```python
from build123d import *

# Parameters (mm, degrees)
SKETCH1_W                       = 25.2476
SKETCH1_H                       = 29.5402
BOSS_EXTRUDE1_DEPTH             = 7.9502
CHAMFER1_SIZE                   = 0.762
CUT_EXTRUDE1_DEPTH              = 30.5402
F_4_40_TAPPED_HOLE1_D           = 2.2606
F_4_40_TAPPED_HOLE1_DEPTH       = 9.5504
F_4_40_TAPPED_HOLE1_CSINK_D     = 4.1148
F_4_40_TAPPED_HOLE1_CSINK_ANGLE = 90
F_4_40_TAPPED_HOLE1_TIP         = 0.679152758
SKETCH6_R                       = 1.6256
SKETCH6_W                       = 3.2512
SKETCH6_H                       = 12.7
CUT_EXTRUDE3_DEPTH              = 8.9502
CUT_EXTRUDE4_DEPTH              = 3.6322
SKETCH11_R                      = 0.635
CUT_EXTRUDE5_DEPTH              = 8.9502
CUT_EXTRUDE7_DEPTH              = 13.6238
CUT_EXTRUDE7_DEPTH_BACK         = 13.6238


with BuildPart() as part:
    # Sketch1 → Boss-Extrude1 (new body)
    with BuildSketch(Plane.XY):
        Rectangle(SKETCH1_W, SKETCH1_H)
    extrude(amount=BOSS_EXTRUDE1_DEPTH)

    # Chamfer1
    chamfer1_edges = [part.edges().sort_by_distance(p)[0] for p in [
        (12.6238, -14.7701, 3.9751),
        (-12.6238, -14.7701, 3.9751),
        (-12.6238, 14.7701, 3.9751),
        (12.6238, 14.7701, 3.9751),
    ]]
    chamfer(chamfer1_edges, length=CHAMFER1_SIZE)

    # Sketch2 → Cut-Extrude1 (cut, through all)
    with BuildSketch(Plane(origin=(0, 14.7701, 0), x_dir=(1, 0, 0), z_dir=(0, 1, 0))):
        Polygon((-6.35, 0.508), (-6.858, 0), (-6.35, -0.508), (-5.842, 0), align=None)
        Polygon((5.842, 0), (6.35, -0.508), (6.858, 0), (6.35, 0.508), align=None)
    extrude(amount=-CUT_EXTRUDE1_DEPTH, mode=Mode.SUBTRACT)

    # #4-40 Tapped Hole1
    with Locations(Plane(origin=(0, 14.7701, 0), x_dir=(1, 0, 0), z_dir=(0, 1, 0))):
        with Locations((-8.89, -3.81), (8.89, -3.81)):
            CounterSinkHole(F_4_40_TAPPED_HOLE1_D / 2, F_4_40_TAPPED_HOLE1_CSINK_D / 2, depth=F_4_40_TAPPED_HOLE1_DEPTH, counter_sink_angle=F_4_40_TAPPED_HOLE1_CSINK_ANGLE)
            with Locations((0, 0, -(F_4_40_TAPPED_HOLE1_DEPTH + F_4_40_TAPPED_HOLE1_TIP / 2))):  # 118° drill point
                Cone(0, F_4_40_TAPPED_HOLE1_D / 2, F_4_40_TAPPED_HOLE1_TIP, mode=Mode.SUBTRACT)

    # Sketch6 → Cut-Extrude3 (cut, through all)
    with BuildSketch(Plane.XY.offset(7.9502)):
        with Locations((-6.35, 0.6985)):
            Circle(SKETCH6_R)
        with Locations((-6.35, -12.0015)):
            Circle(SKETCH6_R)
        with Locations((6.35, -12.0015)):
            Circle(SKETCH6_R)
        with Locations((6.35, 0.6985)):
            Circle(SKETCH6_R)
        with Locations((-6.35, -5.6515)):
            Rectangle(SKETCH6_W, SKETCH6_H)
        with Locations((6.35, -5.6515)):
            Rectangle(SKETCH6_W, SKETCH6_H)
    extrude(amount=-CUT_EXTRUDE3_DEPTH, mode=Mode.SUBTRACT)

    # Sketch8 → Cut-Extrude4 (cut)
    with BuildSketch(Plane.XY.offset(7.9502)):
        with BuildLine():
            ThreePointArc((8.89, 0.6985), (6.35, 3.2385), (3.81, 0.6985))
            Line((3.81, 0.6985), (3.81, -12.0015))
            ThreePointArc((3.81, -12.0015), (6.35, -14.5415), (8.89, -12.0015))
            Line((8.89, -12.0015), (8.89, 0.6985))
        make_face()
        with BuildLine():
            Line((4.7244, -12.0015), (4.7244, 0.6985))
            ThreePointArc((4.7244, 0.6985), (6.35, 2.3241), (7.9756, 0.6985))
            Line((7.9756, 0.6985), (7.9756, -12.0015))
            ThreePointArc((7.9756, -12.0015), (6.35, -13.6271), (4.7244, -12.0015))
        make_face(mode=Mode.SUBTRACT)
        with BuildLine():
            Line((-3.81, -12.0015), (-3.81, 0.6985))
            ThreePointArc((-3.81, 0.6985), (-6.35, 3.2385), (-8.89, 0.6985))
            Line((-8.89, 0.6985), (-8.89, -12.0015))
            ThreePointArc((-8.89, -12.0015), (-6.35, -14.5415), (-3.81, -12.0015))
        make_face()
        with BuildLine():
            ThreePointArc((-7.9756, 0.6985), (-6.35, 2.3241), (-4.7244, 0.6985))
            Line((-4.7244, 0.6985), (-4.7244, -12.0015))
            ThreePointArc((-4.7244, -12.0015), (-6.35, -13.6271), (-7.9756, -12.0015))
            Line((-7.9756, -12.0015), (-7.9756, 0.6985))
        make_face(mode=Mode.SUBTRACT)
    extrude(amount=-CUT_EXTRUDE4_DEPTH, mode=Mode.SUBTRACT)

    # Sketch11 → Cut-Extrude5 (cut, through all)
    with BuildSketch(Plane.XY.offset(7.9502)):
        with Locations((-8.89, 5.8674)):
            Circle(SKETCH11_R)
        with Locations((8.89, 5.8674)):
            Circle(SKETCH11_R)
    extrude(amount=-CUT_EXTRUDE5_DEPTH, mode=Mode.SUBTRACT)

    # Sketch15 → Cut-Extrude7 (cut, two sides)
    with BuildSketch(Plane(origin=(0, 0, 0), x_dir=(0, 0, -1), z_dir=(1, 0, 0))) as cut_extrude7_sk:
        Polygon((-53.679236414, 64.131336414), (-4.318, 14.7701), (-3.81, 14.2621), (-3.302, 14.7701), (46.059236414, 64.131336414), (46.059236414, 203.745996399), (-53.679236414, 203.745996399), align=None)
    extrude(amount=CUT_EXTRUDE7_DEPTH, mode=Mode.SUBTRACT)
    extrude(cut_extrude7_sk.sketch, amount=-CUT_EXTRUDE7_DEPTH_BACK, mode=Mode.SUBTRACT)


solid = part.part
```
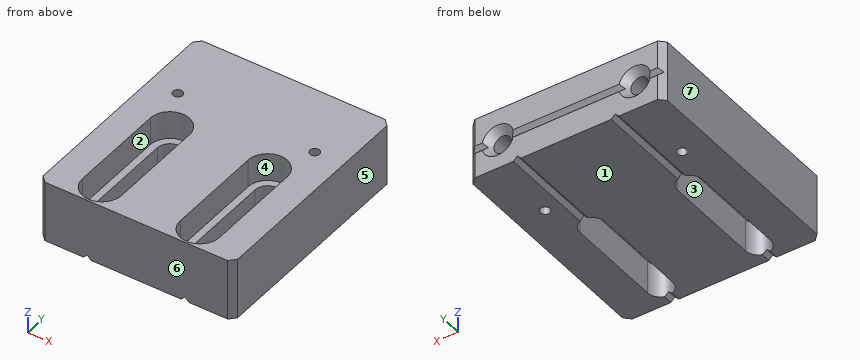
The listing builds one solid part. Answer for the finished solid, in the listing's coordinates (mm). Face numbers are marked on the shaded views. A direction names the side the tool comes from. Coordinates: 2 decimals unless noted, no trailing zeros. Loops run counter-clockwise (first coordinate to the right, second up) from the corner with the lowest first, then second, coordinate; pieces in that order, holes last. Notation, with made-up numbers: (-22.5, 2) -> (14.5, 2) arc R15 ccw to (14.5, 23) -> close; hole circle Ø9 at (-38, 3). An arc over 180 degrees is marked (long way). Return JSON: item names as keys, results as strings. Group by question number.
(1) A cutting plane is placed at C-C on x = -5.25. Write down the section's boundary in (y, z).
(2) Which of the six approach directions +Z, -Z, +X, -X, +Y, -Y give full straight-line access (tool end or side, diameter ignored) to the marked faces 1, 2 and 3?
(3) A cutting plane is placed at B-B on y = -6.25. Write down the section's boundary in (x, z).
(4) Determine the mould class of the marked faces 4, 5, 6 and 7 for opening direction X: released by +X, released by -X, zero draft, split by the parting line, or undercut.
(5) A cutting plane is placed at A-A on y = 9.25. Write down the section's boundary in (x, z).
(6) Given pin 1 Ø1.5 at (x, y) = (-2.5, -6) entering from -Z; pin 2 Ø1.4 at (x, z) = (-8.89, 3.81) entering from +Y, each flat-ended and moving along its own axis, determine where each tip first touches the part or whether it passes through.
(7) Find the intervals of material crossed by probe 1 along X at (y, z) = (0.75, 2.5); probe 2 along X at (y, z) = (-2.75, 7.25); probe 3 along Z at (x, y) = (8.89, 11), in increasing order. Write a range as from..to.
The answers:
{
 "1": {"outline": "(-14.77, 0) -> (-13.2, 0) -> (-13.2, 4.32) -> (-14.29, 4.32) -> (-14.29, 7.95) -> (-14.77, 7.95) -> close; (1.9, 0) -> (14.77, 0) -> (14.77, 3.3) -> (14.26, 3.81) -> (14.77, 4.32) -> (14.77, 7.95) -> (2.99, 7.95) -> (2.99, 4.32) -> (1.9, 4.32) -> close"},
 "2": {"face 1": "-Z, +X, -X, +Y, -Y", "face 2": "+Z", "face 3": "+Z, -Z"},
 "3": {"outline": "(-12.62, 0) -> (-7.98, 0) -> (-7.98, 4.32) -> (-8.89, 4.32) -> (-8.89, 7.95) -> (-12.62, 7.95) -> close; (-4.72, 0) -> (4.72, 0) -> (4.72, 4.32) -> (3.81, 4.32) -> (3.81, 7.95) -> (-3.81, 7.95) -> (-3.81, 4.32) -> (-4.72, 4.32) -> close; (7.98, 0) -> (12.62, 0) -> (12.62, 7.95) -> (8.89, 7.95) -> (8.89, 4.32) -> (7.98, 4.32) -> close"},
 "4": {"face 4": "undercut", "face 5": "released by +X", "face 6": "zero draft", "face 7": "released by -X"},
 "5": {"outline": "(-12.62, 0) -> (-6.86, 0) -> (-6.35, 0.51) -> (-5.84, 0) -> (5.84, 0) -> (6.35, 0.51) -> (6.86, 0) -> (12.62, 0) -> (12.62, 7.95) -> (-12.62, 7.95) -> close; hole circle Ø2.26 at (-8.89, 3.81); hole circle Ø2.26 at (8.89, 3.81)"},
 "6": {"pin 1": "stops at z = 0", "pin 2": "stops at y = 4.96"},
 "7": {"probe 1": "x = -12.62..-7.97, -4.73..4.73, 7.97..12.62", "probe 2": "x = -12.62..-8.89, -3.81..3.81, 8.89..12.62", "probe 3": "z = 0..2.68, 4.94..7.95"}
}
